from build123d import *

# Parameters (mm, degrees)
F1_DEPTH = 15


with BuildPart() as f1:
    # F0 (on Top) → F1 (new body)
    with BuildSketch(Plane.XY):
        with BuildLine():
            Line((30, 10), (-30, 10))
            ThreePointArc((-30, 10), (-37.0710678119, 7.0710678119), (-40, 0))
            ThreePointArc((-40, 0), (-37.0710678119, -7.0710678119), (-30, -10))
            Line((-30, -10), (30, -10))
            add(Edge.make_bspline(
                [(30, -10), (30.4419813549, -9.9690694458), (30.8687106597, -9.941549094), (31.2810670558, -9.9176039041)],
                knots=[0, 0, 0, 0, 0.775534817, 0.775534817, 0.775534817, 0.775534817], degree=3))
            ThreePointArc((31.2810670558, -9.9176039041), (37.51034856, -6.6026255768), (40, 4.32e-08))
            ThreePointArc((40, 4.32e-08), (37.5103485315, 6.6026256092), (31.2810670558, 9.9176039041))
            add(Edge.make_bspline(
                [(30, 10), (30.4419813549, 9.9690694458), (30.8687106597, 9.941549094), (31.2810670558, 9.9176039041)],
                knots=[0, 0, 0, 0, 0.775534817, 0.775534817, 0.775534817, 0.775534817], degree=3))
        make_face()
        with BuildLine():
            Line((30, -5), (-30, -5))
            ThreePointArc((-30, -5), (-35, 0), (-30, 5))
            Line((-30, 5), (30, 5))
            ThreePointArc((30, 5), (35, 0), (30, -5))
        make_face(mode=Mode.SUBTRACT)
        with BuildLine():
            ThreePointArc((-40, 0), (-37.0710678119, 7.0710678119), (-30, 10))
            add(Edge.make_bspline(
                [(-30, 10), (-36.5690253675, 10.6094982475), (-39.7284552455, 10.459353216), (-45.5274550985, 17.3520761307)],
                knots=[0, 0, 0, 0, 17.1800723301, 17.1800723301, 17.1800723301, 17.1800723301], degree=3))
            ThreePointArc((-45.5274550985, 17.3520761307), (-41.4152457852, 9.1055931426), (-40, 0))
        make_face()
        with BuildLine():
            ThreePointArc((-45.5274550985, -17.3520761307), (-41.4152457852, -9.1055931426), (-40, 0))
            ThreePointArc((-40, 0), (-41.4152457852, 9.1055931426), (-45.5274550985, 17.3520761307))
            ThreePointArc((-45.5274550985, 17.3520761307), (-100, 0), (-45.5274550985, -17.3520761307))
        make_face()
        Polygon((-93.0940107676, 0), (-81.5470053838, 20), (-58.4529946162, 20), (-46.9059892324, 0), (-58.4529946162, -20), (-81.5470053838, -20), align=None, mode=Mode.SUBTRACT)
        with BuildLine():
            ThreePointArc((-30, -10), (-37.0710678119, -7.0710678119), (-40, 0))
            ThreePointArc((-40, 0), (-41.4152457852, -9.1055931426), (-45.5274550985, -17.3520761307))
            add(Edge.make_bspline(
                [(-30, -10), (-36.5690253675, -10.6094982475), (-39.7284552455, -10.459353216), (-45.5274550985, -17.3520761307)],
                knots=[0, 0, 0, 0, 17.1800723301, 17.1800723301, 17.1800723301, 17.1800723301], degree=3))
        make_face()
        with BuildLine():
            add(Edge.make_bspline(
                [(31.2810670558, 9.9176039041), (39.496869131, 9.4405191711), (42.0070999801, 10.3826559201), (45.765051322, 14.0487094117)],
                knots=[0.775534817, 0.775534817, 0.775534817, 0.775534817, 16.2273154098, 16.2273154098, 16.2273154098, 16.2273154098], degree=3))
            ThreePointArc((31.2810670558, 9.9176039041), (37.5103485315, 6.6026256092), (40, 4.32e-08))
            ThreePointArc((40, 4.32e-08), (41.4973113717, 7.5927935257), (45.765051322, 14.0487094117))
        make_face()
        with BuildLine():
            ThreePointArc((45.765051322, -14.0487094117), (41.4973113553, -7.5927934857), (40, 4.32e-08))
            ThreePointArc((40, 4.32e-08), (37.51034856, -6.6026255768), (31.2810670558, -9.9176039041))
            add(Edge.make_bspline(
                [(31.2810670558, -9.9176039041), (39.496869131, -9.4405191711), (42.0070999801, -10.3826559201), (45.765051322, -14.0487094117)],
                knots=[0.775534817, 0.775534817, 0.775534817, 0.775534817, 16.2273154098, 16.2273154098, 16.2273154098, 16.2273154098], degree=3))
        make_face()
        with BuildLine():
            ThreePointArc((45.765051322, 14.0487094117), (41.4973113717, 7.5927935257), (40, 4.32e-08))
            ThreePointArc((40, 4.32e-08), (41.4973113553, -7.5927934857), (45.765051322, -14.0487094117))
            add(Edge.make_bspline(
                [(45.765051322, -14.0487094117), (45.8848721077, -14.1656000709), (46.0059613608, -14.2852599399), (46.1285444707, -14.4077313099)],
                knots=[16.2273154098, 16.2273154098, 16.2273154098, 16.2273154098, 16.7199892956, 16.7199892956, 16.7199892956, 16.7199892956], degree=3))
            ThreePointArc((46.1285444707, -14.4077313099), (67.828502073, -18.4041993929), (80, 0))
            ThreePointArc((80, 0), (67.828502073, 18.4041993929), (46.1285444707, 14.4077313099))
            add(Edge.make_bspline(
                [(45.765051322, 14.0487094117), (45.8848721077, 14.1656000709), (46.0059613608, 14.2852599399), (46.1285444707, 14.4077313099)],
                knots=[16.2273154098, 16.2273154098, 16.2273154098, 16.2273154098, 16.7199892956, 16.7199892956, 16.7199892956, 16.7199892956], degree=3))
        make_face()
        Polygon((45.7341522556, 4.6352549156), (60, 15), (74.2658477444, 4.6352549156), (68.8167787844, -12.1352549156), (51.1832212156, -12.1352549156), align=None, mode=Mode.SUBTRACT)
    extrude(amount=F1_DEPTH)


solid = f1.part
Work out the finished part from the listing and answer in its coordinate system (mm). A direction names the side the tool comes from. Round coordinates to 2 decimals unless told otherwise and drop trailing zeros. Order: outer loops, then holes, each group sorted by start corner. A loop starts at its lowest first (then second) coordinate and runs counter-clockwise, first axis right, second up. Notation, with made-up numbers: M 75,37 L 95,37 A22 ccw 95,67 Z; hole C -24.75,14 d8. An arc over 180 degrees is marked long. One line per item, written item: value.
Q1. Find section D-D on x = -70. Write down the section's boundary in (y, z).
Derived:
outline: M -30,0 L -20,0 L -20,15 L -30,15 Z; M 20,0 L 30,0 L 30,15 L 20,15 Z
Q2. Find section B-B on y = 8. Write down the section's boundary in (x, z), then the cut area to 3 significant figures.
Derived:
outline: M -98.91,0 L -88.48,0 L -88.48,15 L -98.91,15 Z; M -51.52,0 L 50.37,0 L 50.37,15 L -51.52,15 Z; M 69.63,0 L 78.33,0 L 78.33,15 L 69.63,15 Z
area: 1,820 mm²
Q3. Straight lines are drawn through the part: line 1 (Y direction, x = -2, z = 6); line 2 (X direction, y = -15.5, z = 12.75); line 3 (X direction, y = -9, z = 7.5). For each, find the intervals that lie inside material, in ascending order.
Derived:
line 1: -10 to -5, 5 to 10
line 2: -95.69 to -84.15, -55.85 to -43.87, 47.36 to 72.64
line 3: -98.62 to -87.9, -52.1 to 50.16, 69.84 to 77.86
Q4. Find section C-C on z = 3.75. Give the number of separate pieces and of enclosed holes in the cut face, then the cut area to 3 significant figures.
Derived:
separate pieces: 1
enclosed holes: 3
area: 3,150 mm²
Q5. Find section A-A on x = 6.5. Write down the section's boundary in (y, z).
Derived:
outline: M -10,0 L -5,0 L -5,15 L -10,15 Z; M 5,0 L 10,0 L 10,15 L 5,15 Z
Q6. Flat-ended cylindrical pins translate along their axes: pin 1 (7.5 mm diameter, centred on x = 1, z = 6, fed in from -Y); pin 2 (6 mm diameter, centred on x = -72.5, z = 5, fed in from +Y); pin 3 (3 mm diameter, centred on x = -59, z = 8, fed in from +Y); pin 4 (4 mm diameter, centred on y = -3.5, z = 4, fed in from +X). Find the tip coordinate at first contact, or state that the pin passes through.
Derived:
pin 1: y = -10
pin 2: y = 30
pin 3: y = 28.46
pin 4: x = 79.94
Q7. Determine the mould class of faces 4 (the face through (71.58, -3.63, 7.4)), 5 (the face through (-99.98, 1.06, 7.4)), 6 (the face through (0, 10, 7)) for opening direction Y: released by +Y, released by -Y, zero draft, split by the parting line, or undercut.
Derived:
face 4: undercut
face 5: split by the parting line
face 6: released by +Y
Q8. For faces 1 (the face through (0, -10, 7)), 2 (the face through (-87.4, 9.86, 7.4)), 3 (the face through (-17, 7, 15)), determine the directions among +Z, -Z, +X, -X, +Y, -Y from which every point of the face is accessible in a straight line to the end or side of a thin tool.
Derived:
face 1: +Z, -Z, -Y
face 2: +Z, -Z
face 3: +Z, +X, -X, +Y, -Y
